Part model, mm, in its own coordinate system. Face numbers are marked on the shaded views. A direction names the side the tool comes from. Round coordinates to 2 decimals unless told otherwise and drop trailing zeros. Loops run counter-clockwise (first coordinate to the right, second up) from the corner with the lowest first, then second, coordinate; pieces in that order, holes last. Notation, with made-up numbers: M -17.5,80 L 38.5,80 A20 ccw 38.5,112 Z; hole C 2,-28.75 d11. An arc over 180 degrees is marked long. Answer as CSV lines item,"result". Start each with the question number.
Item 1: Which spindle directions (+Z, -Z, +X, -X, +Y, -Y) get a long thin tool onto all of the face, cutting with end or side? Do the marked faces 1, 2, 3, 4 and 5. Say none if no direction does.
Item 2: Band-saw the part on D-D (x = 6.25). Give the cut face in (y, z).
Item 3: Wall check: line 1 (Z direction, x = 8.75, y = -2.5); line 2 (Z direction, x = -2.5, y = 1.5); line 3 (X direction, y = -0.5, z = 9). Give the ranges that are in metal, low to high.
Item 4: Drop flat-ended pins along their axis: pin 1 Ø1.5 at (y, z) = (-2, 8.5) entering from -X; pin 2 Ø2.5 at (x, y) = (-4.11, 0) entering from +Z; pin 3 Ø0.9 at (x, y) = (9, -2) entering from +Z; pin 4 Ø5 at (x, z) = (-5, 8) entering from -Y. Give the stop position or say it passes through.
Item 5: Band-saw the part on B-B (z = 4.5). Give the cut face in (x, y), and give its area (3 significant figures).
Item 6: Band-saw the part on A-A (z = 1.5). Count the separate pieces of the cut face and the enclosed holes in it, and give its area (3 significant figures).
```python
from build123d import *

# Parameters (mm, degrees)
F0_W      = 18
F0_H      = 6
F1_DEPTH  = 2
F2_R      = 3
F2_R_2    = 2
F3_DEPTH  = 10
F4_R      = 1
F4_R_2    = 1.15
F5_DEPTH  = 20
F6_SIZE2  = 1.5
F6_SIZE   = 0.6
F7_W      = 11.6012076614
F7_H      = 11.8295210414
F8_DEPTH  = 7
F9_R      = 2.9999
F10_R     = 1.9
F10_R_2   = 1
F11_DEPTH = 3


# Not quite as in the source:
# - a fillet or chamfer is up to 0.001 mm smaller than in the source, because OpenCascade refuses the exact size


with BuildPart() as f1:
    # F0 (on Top) → F1 (new body)
    with BuildSketch(Plane.XY):
        with Locations((1.8924829921, 0)):
            Rectangle(F0_W, F0_H)
    extrude(amount=F1_DEPTH)

    # F2 (on face) → F3 (join)
    with BuildSketch(Plane.XY.offset(2)):
        with Locations((7.8924829921, 0)):
            Circle(F2_R)
        with Locations((-4.1075170079, 0)):
            Circle(F2_R_2)
    extrude(amount=F3_DEPTH)

    # F4 (on face) → F5 (cut)
    with BuildSketch(Plane.XY.offset(12)):
        with Locations((-4.1075170079, 0)):
            Circle(F4_R)
        with Locations((7.8924829921, 0)):
            Circle(F4_R_2)
    extrude(amount=-F5_DEPTH, mode=Mode.SUBTRACT)

    # F6
    f6_edges = [f1.edges().sort_by_distance(p)[0] for p in [
        (-6.107517, 0, 12),
    ]]
    f6_side = f1.faces().sort_by_distance((-6.050948, 0, 12))[0]
    chamfer(f6_edges, length=F6_SIZE, length2=F6_SIZE2, reference=f6_side)

    # F7 (on face) → F8 (cut)
    with BuildSketch(Plane.XY.offset(12)):
        with Locations((7.5882198871, -0.5373002496)):
            Rectangle(F7_W, F7_H)
    extrude(amount=-F8_DEPTH, mode=Mode.SUBTRACT)

    # F9 (radius 3 in the source; OpenCascade refuses exactly that, so slightly less here)
    f9_edges = [f1.edges().sort_by_distance(p)[0] for p in [
        (10.892483, -3, 1),
        (10.892483, 3, 1),
        (-7.107517, 3, 1),
        (-7.107517, -3, 1),
    ]]
    fillet(f9_edges, radius=F9_R)

    # F10 (on face) → F11 (join)
    with BuildSketch(Plane(origin=(0, 0, 0), x_dir=(1, 0, 0), z_dir=(0, 0, -1))):
        with Locations((-4.1075170079, 0)):
            Circle(F10_R)
        with Locations((-4.1075170079, 0)):
            Circle(F10_R_2, mode=Mode.SUBTRACT)
    extrude(amount=F11_DEPTH)


solid = f1.part
```
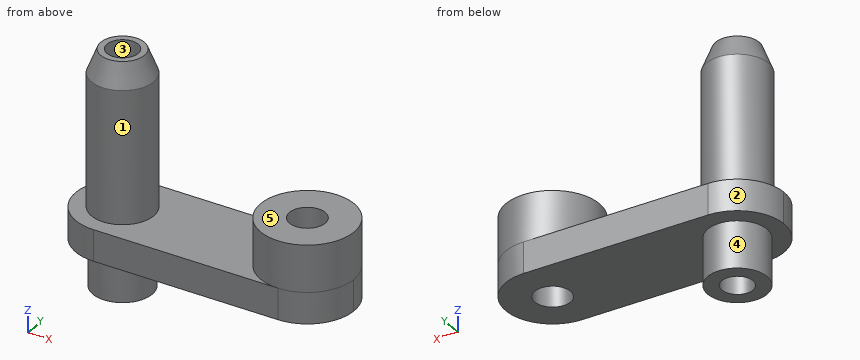
Answer block:
1,face 1,"+Z"
1,face 2,"+Z, -Z, -X, +Y"
1,face 3,"+Z, -Z"
1,face 4,"-Z"
1,face 5,"+Z, +X, +Y, -Y"
2,outline,"M -3,0 L 3,0 L 3,2 L 2.51,2 L 2.51,5 L -2.51,5 L -2.51,2 L -3,2 Z"
3,line 1,"z = 0 to 5"
3,line 2,"z = 0 to 2"
3,line 3,"x = -6.04 to -4.97, -3.24 to -2.17"
4,pin 1,"stops at x = -5.67"
4,pin 2,"stops at z = 12"
4,pin 3,"stops at z = 5"
4,pin 4,"stops at y = -2"
5,outline,"C -4.11,0 d4; C 7.89,0 d6; hole C -4.11,0 d2; hole C 7.89,0 d2.3"
5,area,"33.5 mm^2"
6,separate pieces,"1"
6,enclosed holes,"2"
6,area,"93.0 mm^2"
